Autodesk Inventor part; units mm, degrees
ref_plane "YZ Plane" through (0, 0, 0) normal (1, 0, 0) x (0, 1, 0)
ref_plane "XZ Plane" through (0, 0, 0) normal (0, 1, 0) x (-1, 0, 0)
ref_plane "XY Plane" through (0, 0, 0) normal (0, 0, 1) x (1, 0, 0)
sketch "スケッチ1" plane through (0, 0, 0) normal (1, 0, 0) x (0, 1, 0)
  arc A0 (8.4759, 50) -> (8.4759, -50) centre (234.0113, 0) ccw
  arc A1 (5.547, 50.6493) -> (5.547, -50.6493) centre (234.0113, 0) ccw
  line L0 (8.4759, 50) -> (5.547, 50.6493)
  line L1 (8.4759, -50) -> (5.547, -50.6493)
  line L2 (0, -70.909) -> (0, 70.909)
  point P0 (0, 0)
  point P1 (0, 0)
  dimension "d0" = 3
  dimension "d1" = 100
  dimension "d2" = 25
extrude "押し出し1" add sketch "スケッチ1" along normal blind 200
sketch "スケッチ2" plane through (0, 0, 0) normal (-1, 0, 0) x (0, 0, 1)
  line L0 (-50.6493, 5.547) -> (-50, 8.4759)
  line L1 (-50.5452, 6.0168) -> (-35.9007, 2.7702)
  arc A0 (-50.6493, 5.547) -> (50.6493, 5.547) centre (0, 234.0113) ccw
  line L2 (-50, 8.4759) -> (-50.6493, 5.547)
  point P0 (0, 0)
  dimension "d5" = 15
extrude "押し出し2" cut sketch "スケッチ2" against normal through all
mirror "ミラー1" about plane through (0, 0, 0) normal (0, 0, 1) of "押し出し2"
properties part number "element_1" material "CFRP"
The model under review builds one solid part; all positions refer to its coordinate system, in mm. Round coordinates to 2 decimals unless told otherwise and drop trailing zeros. Order: outer loops, then holes, each group sorted by start corner. A loop starts at its lowest first (then second) coordinate and runs counter-clockwise, first axis right, second up.
Item 1: Add section A-A, the plane x = 185.5. State the section outline as (y, z) points.
Working result:
outline: (2.77, -35.9) - (6.02, -50.55) - (8.48, -50) arc R231.01 cw to (8.48, 50) - (6.02, 50.55) - (2.77, 35.9) arc R234.01 ccw to start
Item 2: For pin 1 (1 mm diameter, centred on x = 103, z = -2.5, fed in from -Y); pin 2 (5 mm diameter, centred on x = 146.5, y = 5, fed in from +Z); pin 3 (12 mm diameter, centred on x = 80.5, z = -3, fed in from +Y), all flat-tipped, find the tip position at first contact; note any pin that passes through.
Working result:
pin 1: stops at y = 0.01
pin 2: stops at z = 50.55
pin 3: stops at y = 3.18
Item 3: Add section C-C, the plane z = -7. State the section outline as (x, y) points, and give its area (3 significant figures).
Working result:
outline: (0, 0.1) - (200, 0.1) - (200, 3.11) - (0, 3.11) - close
area: 600 mm2
Item 4: To check wall thickness, follow probe 1 along Y at (x, z) = (56, -2); probe 2 along Y at (x, z) = (16.5, 28). State the ranges of each line that lie inside material, in increasing order.
Working result:
probe 1: y = 0.01 to 3.01
probe 2: y = 1.68 to 4.7
Item 5: Draft analysis for pull direction Z (two halves, no side actions). For faces 1 (the flat face through (98.6, 4.416, -43.325)), 2 (the cylindrical face through (98.6, 0, -0.5)), 3 (the cylindrical face through (98.6, 3, -0.7)), state which applies: released by +Z, released by -Z, zero draft, split by the parting line, or undercut.
Working result:
face 1: released by -Z
face 2: split by the parting line
face 3: undercut
